from build123d import *

# Parameters (mm, degrees)
SKETCH1_R           = 152.4
SKETCH1_R_2         = 2.070099999999984
SKETCH1_R_3         = 2.0700999999999827
SKETCH1_R_4         = 2.070099999999987
SKETCH1_R_5         = 2.0700999999999805
SKETCH1_R_6         = 2.070099999999982
SKETCH1_R_7         = 2.070099999999981
SKETCH1_R_8         = 2.07009999999998
SKETCH1_R_9         = 2.0700999999999787
SKETCH1_R_10        = 2.070099999999999
SKETCH1_R_11        = 2.070099999999978
SKETCH1_R_12        = 2.0700999999999765
SKETCH1_R_13        = 2.0700999999999934
SKETCH1_R_14        = 2.0700999999999747
BOSS_EXTRUDE1_DEPTH = 2.286
CUT_EXTRUDE1_DEPTH  = 216.53826991047322
CIRPATTERN1_COUNT   = 8
FILLET1_R           = 6.35


with BuildPart() as part:
    # Sketch1 → Boss-Extrude1 (new body)
    with BuildSketch(Plane(origin=(0, 0, 0), x_dir=(1, 0, 0), z_dir=(0, 1, 0))):
        with Locations(Location((0, 0, 0), (0, 0, 270))):
            Circle(SKETCH1_R)
        with Locations(Location((-143.9799, 1.749e-14, 0), (0, 0, 270))):
            Circle(SKETCH1_R_2, mode=Mode.SUBTRACT)
        with Locations(Location((-124.9299, -1.53e-14, 0), (0, 0, 270))):
            Circle(SKETCH1_R_3, mode=Mode.SUBTRACT)
        with Locations(Location((-101.8091636445608, 101.80916364456118, 0), (0, 0, 270))):
            Circle(SKETCH1_R_4, mode=Mode.SUBTRACT)
        with Locations(Location((-88.33877946295712, 88.33877946295739, 0), (0, 0, 270))):
            Circle(SKETCH1_R_5, mode=Mode.SUBTRACT)
        with Locations(Location((5.202e-13, 143.9799, 0), (0, 0, 270))):
            Circle(SKETCH1_R_6, mode=Mode.SUBTRACT)
        with Locations(Location((4.2089e-13, 124.9299, 0), (0, 0, 270))):
            Circle(SKETCH1_R_7, mode=Mode.SUBTRACT)
        with Locations(Location((101.80916364456154, 101.80916364456044, 0), (0, 0, 270))):
            Circle(SKETCH1_R_4, mode=Mode.SUBTRACT)
        with Locations(Location((88.3387794629577, 88.33877946295681, 0), (0, 0, 270))):
            Circle(SKETCH1_R_5, mode=Mode.SUBTRACT)
        with Locations(Location((143.9799, -1.0229e-12, 0), (0, 0, 270))):
            Circle(SKETCH1_R_8, mode=Mode.SUBTRACT)
        with Locations(Location((124.9299, -8.5708e-13, 0), (0, 0, 270))):
            Circle(SKETCH1_R_9, mode=Mode.SUBTRACT)
        with Locations(Location((101.8091636445601, -101.80916364456186, 0), (0, 0, 270))):
            Circle(SKETCH1_R_10, mode=Mode.SUBTRACT)
        with Locations(Location((88.33877946295651, -88.33877946295799, 0), (0, 0, 270))):
            Circle(SKETCH1_R_4, mode=Mode.SUBTRACT)
        with Locations(Location((-1.5256e-12, -143.9799, 0), (0, 0, 270))):
            Circle(SKETCH1_R_11, mode=Mode.SUBTRACT)
        with Locations(Location((-1.29327e-12, -124.9299, 0), (0, 0, 270))):
            Circle(SKETCH1_R_12, mode=Mode.SUBTRACT)
        with Locations(Location((-101.80916364456223, -101.80916364455973, 0), (0, 0, 270))):
            Circle(SKETCH1_R_13, mode=Mode.SUBTRACT)
        with Locations(Location((-88.3387794629583, -88.3387794629562, 0), (0, 0, 270))):
            Circle(SKETCH1_R_14, mode=Mode.SUBTRACT)
    extrude(amount=BOSS_EXTRUDE1_DEPTH)

    # Sketch2 → Cut-Extrude1 (cut, through all)
    with BuildSketch(Plane(origin=(0, 2.286, 0), x_dir=(1, 0, 0), z_dir=(0, 1, 0))):
        with BuildLine():
            ThreePointArc((3.1750000000002516, -117.13134506911759), (6.986841257319973, -120.23073696228855), (8.420099999998719, -124.9299))
            Line((8.420099999998717, -124.9299), (8.420099999998637, -131.6668670394721))
            ThreePointArc((8.420099999998639, -131.6668670394721), (12.88163120444934, -141.3321467511392), (23.131538095236692, -144.2065686622791))
            ThreePointArc((23.13153809523673, -144.2065686622791), (55.89091529692152, -134.93260572327338), (85.61297514632435, -118.32591003915775))
            ThreePointArc((85.6129751463244, -118.32591003915772), (90.82823058997255, -109.04560814479298), (87.14862473293043, -99.05644434946592))
            Line((87.14862473293043, -99.05644434946592), (82.38486965468944, -94.29268927122504))
            ThreePointArc((82.38486965468765, -94.29268927122683), (80.07552658096357, -89.95641224521594), (80.5793043576061, -85.06943241814194))
            Line((80.57930435760602, -85.069432418142), (14.554814795987514, -19.044942856522383))
            ThreePointArc((14.554814795987514, -19.04494285652238), (11.14164107789032, -17.22056340123132), (7.290119914433424, -17.599904875685596))
            ThreePointArc((7.290119914433424, -17.599904875685596), (4.298447514577617, -20.055106641508246), (3.174999999999997, -23.758616482314267))
            Line((3.174999999999999, -23.758616482314267), (3.175, -117.13134506911767))
        make_face()
    cut_extrude1 = extrude(amount=-CUT_EXTRUDE1_DEPTH, mode=Mode.SUBTRACT)

    # CirPattern1: Cut-Extrude1 ×8 about axis
    cirpattern1_axis = Axis((4.806e-14, 0, -1.941e-14), (0, 1, 0))
    for i in range(1, CIRPATTERN1_COUNT):
        add(cut_extrude1.rotate(cirpattern1_axis, i * 360 / CIRPATTERN1_COUNT), mode=Mode.SUBTRACT)

    # Fillet1
    fillet1_edges = [part.edges().sort_by_distance(p)[0] for p in [
        (117.1313450691169, 1.143, 3.1750000000009777),
        (85.06943241814194, 1.143, 80.57930435760721),
        (-85.06943241814196, 1.143, 80.57930435760598),
        (-117.1313450691176, 1.143, 3.1750000000000322),
        (-3.17500000000097, 1.143, 117.13134506911682),
        (-80.5793043576072, 1.143, 85.06943241814186),
        (-117.13134506911682, 1.143, -3.1750000000010234),
        (-85.06943241814184, 1.143, -80.57930435760727),
        (85.06943241814206, 1.143, -80.57930435760602),
        (117.1313450691177, 1.143, -3.175000000000084),
        (3.175000000001045, 1.143, -117.13134506911688),
        (80.57930435760728, 1.143, -85.06943241814191),
        (-80.57930435760595, 1.143, -85.06943241814203),
        (-3.175000000000016, 1.143, -117.13134506911767),
        (80.57930435760606, 1.143, 85.06943241814197),
        (3.175000000000126, 1.143, 117.13134506911763),
    ]]
    fillet(fillet1_edges, radius=FILLET1_R)


solid = part.part
Geometry check sheet. Reference: the model listing, model coordinates, mm. Coordinates: 2 decimals unless noted, no trailing zeros. Order: outer loops, then holes, each group sorted by start corner. A loop starts at its lowest first (then second) coordinate and runs counter-clockwise, first axis right, second up. Notation, with made-up numbers: (77.5, 24) -> (91.5, 24) arc R18 ccw to (91.5, 38) -> close; hole circle Ø3 at (15, 4.5). An arc over 180 degrees is marked (long way). Use a Markdown table: item, result. Add a question column.
1. Cross-section at B-B (z = -73). Enter the section's corners in (x, y) (3 decimals), and give its area (3 significant figures).
2. Cross-section at C-C (y = 0.6). Give the number of separate pieces and of enclosed holes in the cut face, and give its area (3 significant figures).
3. Go/stop test with flat-tipped pins: pin 1 Ø0.7 at (y, z) = (1.5, -55) entering from -X; pin 2 Ø3.5 at (x, z) = (-143.98, 0) entering from +Y; pin 3 Ø1.1 at (y, z) = (1, 82.5) entering from +X; pin 4 Ø1.1 at (x, y) = (-72.5, 1) entering from -Z. Record where each tip stops, or that it passes through.
4. Material ranges on L1, parallel to X at y = 0.7, z = 0; L2, parallel to Z at x = 57.5, y = 1.75 (1 decimal); L3, parallel to X at y = 0.6, z = 68 (3 decimals), recorded low to high.
5. Cross-section at A-A (x = -34). Enter the section's corners in (y, z) (3 decimals).
6. Mould release check, pull along Z, two halves, no side actions. Record for faces 1 (the face through (2, 2.286, -2)), 2 (the face through (-7.189, 1.159, 17.643)): pulls with the +Z half, pulls with the -Z half, needs draft (parallel to the pull), parting line crosses it, or undercut.
Filled sheet:
| question | item | result |
|---|---|---|
| 1 | outline | (-133.779, 0) -> (-126.497, 0) -> (-126.497, 2.286) -> (-133.779, 2.286) -> close; (-77.49, 0) -> (-68.51, 0) -> (-68.51, 2.286) -> (-77.49, 2.286) -> close; (-3.175, 0) -> (3.175, 0) -> (3.175, 2.286) -> (-3.175, 2.286) -> close; (68.51, 0) -> (77.49, 0) -> (77.49, 2.286) -> (68.51, 2.286) -> close; (126.497, 0) -> (133.779, 0) -> (133.779, 2.286) -> (126.497, 2.286) -> close |
| 1 | area | 88.9 mm2 |
| 2 | separate pieces | 1 |
| 2 | enclosed holes | 24 |
| 2 | area | 16,400 mm2 |
| 3 | pin 1 | x = -142.26 |
| 3 | pin 2 | through |
| 3 | pin 3 | x = 128.49 |
| 3 | pin 4 | z = -134.35 |
| 4 | L1 | -152.4 to -146.05, -141.91 to -127, -122.86 to 122.86, 127 to 141.91, 146.05 to 152.4 |
| 4 | L2 | -141.1 to -134.3, -62 to -53, -3.2 to 3.2, 53 to 62, 134.3 to 141.1 |
| 4 | L3 | -136.388 to -129.254, -72.49 to -63.51, -3.175 to 3.175, 63.51 to 72.49, 129.254 to 136.388 |
| 5 | outline | (0, -148.559) -> (2.286, -148.559) -> (2.286, -142.037) -> (0, -142.037) -> close; (0, -38.49) -> (2.286, -38.49) -> (2.286, -29.51) -> (0, -29.51) -> close; (0, -3.175) -> (2.286, -3.175) -> (2.286, 3.175) -> (0, 3.175) -> close; (0, 29.51) -> (2.286, 29.51) -> (2.286, 38.49) -> (0, 38.49) -> close; (0, 142.037) -> (2.286, 142.037) -> (2.286, 148.559) -> (0, 148.559) -> close |
| 6 | face 1 | needs draft |
| 6 | face 2 | undercut |
